Input: dimensioned drawing with shaded views. Units: mm. Origin: part minimum x, y, z. A direction names the side the tool comes from. Coordinates: 2 decimals unless noted, no trailing zeros. Loops run counter-clockwise (first coordinate to the right, second up) from the corner with the lowest first, then second, coordinate; pieces in that order, holes last. Notation, with made-up numbers: (8.25, 42) -> (12.25, 42) arc R30 ccw to (12.25, 69) -> close; hole circle Ø3 at (50, 40.5). An arc over 180 degrees is marked (long way). Answer as CSV lines item,"result".
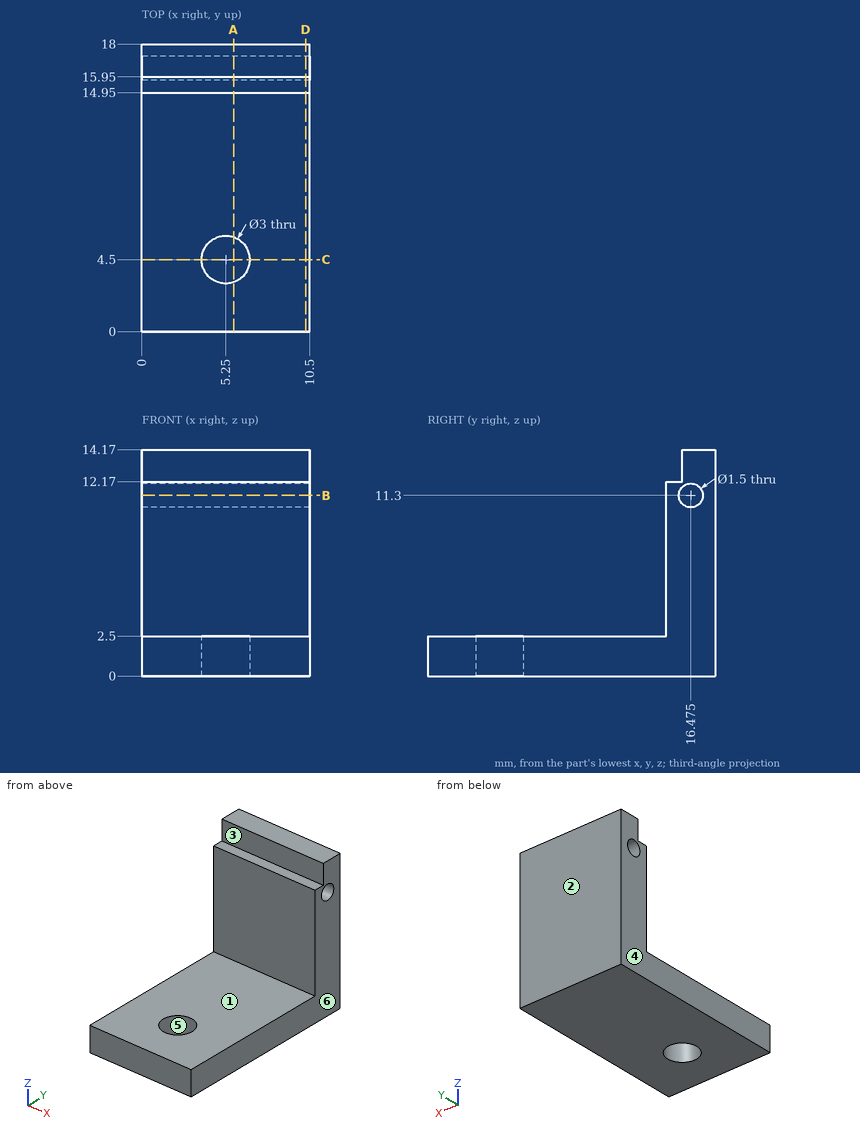
(1) Cut plane A-A (x = 5.75). Return the cut outline in (y, z) (3 decimals), then the cut area to 3 significant figures.
Computed values:
outline,"(0, 0) -> (3.086, 0) -> (3.086, 2.5) -> (0, 2.5) -> close; (5.914, 0) -> (18, 0) -> (18, 14.17) -> (15.95, 14.17) -> (15.95, 12.17) -> (14.95, 12.17) -> (14.95, 2.5) -> (5.914, 2.5) -> close; hole circle Ø1.5 at (16.475, 11.3)"
area,"69.8 mm^2"
(2) Cut plane C-C (y = 4.5). Return the cut outline in (x, z).
Computed values:
outline,"(0, 0) -> (3.75, 0) -> (3.75, 2.5) -> (0, 2.5) -> close; (6.75, 0) -> (10.5, 0) -> (10.5, 2.5) -> (6.75, 2.5) -> close"
(3) Cut plane B-B (z = 11.3). Return the cut outline in (x, y) (3 decimals), then the cut area to 3 significant figures.
Computed values:
outline,"(0, 14.95) -> (10.5, 14.95) -> (10.5, 15.725) -> (0, 15.725) -> close; (0, 17.225) -> (10.5, 17.225) -> (10.5, 18) -> (0, 18) -> close"
area,"16.3 mm^2"
(4) Pin query (flat end, axial travel): pin 1 Ø6 at (x, y) = (5, 3) entering from -Z; pin 2 Ø4 at (x, y) = (6.5, 3) entering from +Z; pin 3 Ø0.6 at (x, z) = (5, 13.5) entering from -Y; pin 4 Ø0.9 at (y, z) = (16.475, 11.3) entering from -X. Return the tip coordinate at first contact, or that it passes through.
Computed values:
pin 1,"z = 0"
pin 2,"z = 2.5"
pin 3,"y = 15.95"
pin 4,"through"
(5) Access query for the marked faces 1 and 2. Directions: +Z, -Z, +X, -X, +Y, -Y. A direction counts if a zero-diameter tool reaches every point of the face in a straight line with its end or side. Return the directions, or none.
Computed values:
face 1,"+Z, +X, -X, -Y"
face 2,"+Z, -Z, +X, -X, +Y"
(6) Cut plane D-D (x = 10.25). Return the cut outline in (y, z) (3 decimals).
Computed values:
outline,"(0, 0) -> (18, 0) -> (18, 14.17) -> (15.95, 14.17) -> (15.95, 12.17) -> (14.95, 12.17) -> (14.95, 2.5) -> (0, 2.5) -> close; hole circle Ø1.5 at (16.475, 11.3)"
(7) Material intervals for L1, parallel to Y at x = 5.75, z = 11.3 (3 decimals); L2, parallel to Z at x = 10.25, y = 13; L3, parallel to Y at x = 6.75, z = 2.75, sorted ascending. Write a range as [from, to].
Computed values:
L1,"[14.95, 15.725], [17.225, 18]"
L2,"[0, 2.5]"
L3,"[14.95, 18]"
(8) Draft query along X for the marked faces 3, 4, 5 and 6. Return one class per face: released by +X, released by -X, zero draft, split by the parting line, or undercut.
Computed values:
face 3,"zero draft"
face 4,"released by -X"
face 5,"undercut"
face 6,"released by +X"
